Design review of the part built by this model. Coordinates are the model's own, in mm. A direction names the side the tool comes from. Give positions to 0.01 mm unless a question says otherwise; leave off trailing zeros. Order: outer loops, then holes, each group sorted by start corner. A loop starts at its lowest first (then second) coordinate and runs counter-clockwise, first axis right, second up.
```python
from build123d import *

# Parameters (mm, degrees)
SKETCH1_R           = 2.4
BOSS_EXTRUDE1_DEPTH = 4
SKETCH2_R           = 3.1
CUT_EXTRUDE1_DEPTH  = 1


with BuildPart() as part:
    # Sketch1 → Boss-Extrude1 (new, symmetric)
    with BuildSketch(Plane.XY):
        with BuildLine():
            Line((-16, -3.5), (16, -3.5))
            ThreePointArc((16, -3.5), (18.474873734, -2.474873734), (19.5, 0))
            Line((19.5, 0), (19.5, 16))
            ThreePointArc((19.5, 16), (16, 19.5), (12.5, 16))
            Line((12.5, 16), (12.5, 3.5))
            Line((12.5, 3.5), (-16, 3.5))
            ThreePointArc((-16, 3.5), (-19.5, 0), (-16, -3.5))
        make_face()
        Circle(SKETCH1_R, mode=Mode.SUBTRACT)
        with Locations((8, 0)):
            Circle(SKETCH1_R, mode=Mode.SUBTRACT)
        with Locations((16, 0)):
            Circle(SKETCH1_R, mode=Mode.SUBTRACT)
        with Locations((-8, 0)):
            Circle(SKETCH1_R, mode=Mode.SUBTRACT)
        with Locations((-16, 0)):
            Circle(SKETCH1_R, mode=Mode.SUBTRACT)
        with Locations((16, 8)):
            Circle(SKETCH1_R, mode=Mode.SUBTRACT)
        with Locations((16, 16)):
            Circle(SKETCH1_R, mode=Mode.SUBTRACT)
    extrude(amount=BOSS_EXTRUDE1_DEPTH, both=True)

    # Sketch2 → Cut-Extrude1 (cut)
    with BuildSketch(Plane.XY.offset(4)):
        with Locations((-16, 0)):
            Circle(SKETCH2_R)
        with Locations((-8, 0)):
            Circle(SKETCH2_R)
        Circle(SKETCH2_R)
        with Locations((8, 0)):
            Circle(SKETCH2_R)
        with Locations((16, 0)):
            Circle(SKETCH2_R)
        with Locations((16, 8)):
            Circle(SKETCH2_R)
        with Locations((16, 16)):
            Circle(SKETCH2_R)
    cut_extrude1 = extrude(amount=-CUT_EXTRUDE1_DEPTH, mode=Mode.SUBTRACT)

    # Mirror1: Cut-Extrude1 across plane
    add(cut_extrude1.mirror(Plane.XY), mode=Mode.SUBTRACT)


solid = part.part
```
1. Take a section at D-D (y = 12). State the section outline as (x, z) points, then the cut area to 3 significant figures.
Recorded:
outline: (12.5, -4) - (19.5, -4) - (19.5, 4) - (12.5, 4) - close
area: 56.0 mm2
2. Take a section at C-C (z = 0). State the section outline as (x, y) points.
Recorded:
outline: (-16, -3.5) - (16, -3.5) arc R3.5 ccw to (19.5, 0) - (19.5, 16) arc R3.5 ccw to (12.5, 16) - (12.5, 3.5) - (-16, 3.5) arc R3.5 ccw to start; hole circle Ø4.8 at (-16, 0); hole circle Ø4.8 at (-8, 0); hole circle Ø4.8 at (0, 0); hole circle Ø4.8 at (8, 0); hole circle Ø4.8 at (16, 0); hole circle Ø4.8 at (16, 8); hole circle Ø4.8 at (16, 16)
3. Machinability: for faces 4 (the face through (12.5, 10, 0)), 5 (the face through (-13.043, 0.931, 3.507)), 6 (the face through (-10.398, 0.106, -0.042)), 7 (the face through (-14, -2, -3)), which of the approach directions +Z, -Z, +X, -X, +Y, -Y give a long, thin tool a straight path to every point of the face, cutting with its end or side? Answer none if there is none.
Recorded:
face 4: +Z, -Z, -X, +Y
face 5: +Z
face 6: +Z, -Z
face 7: -Z
4. Draft analysis for pull direction Y (two halves, no side actions). For faces 1 (the face through (6, 3, -4)), 2 (the face through (18.957, 8.931, -3.507)), 3 (the face through (0, -3.5, 0)), state which applies: pulls with the +Y half, pulls with the -Y half, needs draft (parallel to the pull), parting line crosses it, or undercut.
Recorded:
face 1: needs draft
face 2: undercut
face 3: pulls with the -Y half
5. For line 1 along Y through (x, z) = (8, 1.5); line 2 along Z through (x, y) = (16.5, 2.75); line 3 along Y through (x, z) = (15.5, 1.5), list the stretches that pass through material, from the lowest coordinate up.
Recorded:
line 1: y = -3.5 to -2.4, 2.4 to 3.5
line 2: z = -3 to 3
line 3: y = -3.5 to -2.35, 2.35 to 5.65, 10.35 to 13.65, 18.35 to 19.46
6. For pin 1 (7 mm diameter, centred on x = 17.5, y = 15, fed in from +Z); pin 2 (6 mm diameter, centred on x = 16, y = 8, fed in from -Z); pin 3 (1.9 mm diameter, centred on x = -17.5, y = 1, fed in from +Z), all flat-tipped, find the tip position at first contact; note any pin that passes through.
Recorded:
pin 1: stops at z = 4
pin 2: stops at z = -3
pin 3: stops at z = 3
7. Take a section at A-A (y = 8). State the section outline as (x, z) points.
Recorded:
outline: (12.5, -4) - (12.9, -4) - (12.9, -3) - (13.6, -3) - (13.6, 3) - (12.9, 3) - (12.9, 4) - (12.5, 4) - close; (18.4, -3) - (19.1, -3) - (19.1, -4) - (19.5, -4) - (19.5, 4) - (19.1, 4) - (19.1, 3) - (18.4, 3) - close
8. Take a section at B-B (x = -8). State the section outline as (y, z) points, then the cut area to 3 significant figures.
Recorded:
outline: (-3.5, -4) - (-3.1, -4) - (-3.1, -3) - (-2.4, -3) - (-2.4, 3) - (-3.1, 3) - (-3.1, 4) - (-3.5, 4) - close; (2.4, -3) - (3.1, -3) - (3.1, -4) - (3.5, -4) - (3.5, 4) - (3.1, 4) - (3.1, 3) - (2.4, 3) - close
area: 14.8 mm2
